Read the model definition and answer for the solid it produces. Units are mm, in the model's axes. Give positions to 0.01 mm unless a question says otherwise; leave off trailing zeros. Order: outer loops, then holes, each group sorted by start corner. A loop starts at its lowest first (then second) coordinate and runs counter-clockwise, first axis right, second up. Notation, with made-up numbers: M -11,10.25 L 6,10.25 A33 ccw 6,45.25 Z; hole C 68.5,-2.75 d8. An arc over 180 degrees is marked long. Write item = value, one per line. Start each with the question number.
from build123d import *

# Parameters (mm, degrees)
CROQUIS1_R              = 29.5
CROQUIS1_W              = 10
CROQUIS1_H              = 3
SALIENTE_EXTRUIR1_DEPTH = 3


with BuildPart() as part:
    # Croquis1 → Saliente-Extruir1 (new body)
    with BuildSketch(Plane(origin=(0, 0, 0), x_dir=(0, 0, -1), z_dir=(1, 0, 0))):
        with BuildLine():
            Line((-60, -82), (-40, -82))
            Line((-40, -82), (-40, -85))
            Line((-40, -85), (-20, -85))
            Line((-20, -85), (-20, -82))
            Line((-20, -82), (0, -82))
            Line((0, -82), (0, -85))
            Line((0, -85), (20, -85))
            Line((20, -85), (20, -82))
            Line((20, -82), (40, -82))
            Line((40, -82), (40, -85))
            Line((40, -85), (60, -85))
            Line((60, -85), (60, 25))
            ThreePointArc((60, 25), (0, 85), (-60, 25))
            Line((-60, 25), (-60, -82))
        make_face()
        with Locations((0, 25)):
            Circle(CROQUIS1_R, mode=Mode.SUBTRACT)
        with Locations((15, -60.5)):
            Rectangle(CROQUIS1_W, CROQUIS1_H, mode=Mode.SUBTRACT)
    extrude(amount=SALIENTE_EXTRUIR1_DEPTH)


solid = part.part
1) Find section C-C on y = 35. Determine the outline of the cut face in (x, z), plus the area to 3 significant figures.
2) Find section D-D on y = 71. Determine the outline of the cut face in (x, z).
3) Each of these flat-tipped pins is pushed along its axis until it touches: P1, Ø1.5, axis at x = 2, z = -31.5, coming from the -Y side; P2, Ø0.9, axis at x = 1, y = -83.5, coming from the +Z side. Where does it stop, or does it pass through?
4) Find section B-B on z = -26.5. Determine the outline of the cut face in (x, y), plus the area to 3 significant figures.
5) Find the intervals of material crossed by probe 1 along Y at (x, z) = (2.3, -15); probe 2 along Y at (x, z) = (0.7, -6.5); probe 3 along Y at (x, z) = (2, -2), in increasing order. Write a range as [from, to].
6) Find section A-A on x = 1.55. Determine the outline of the cut face in (y, z).
7) For a pull along Y with two mould halves and no side action, classify faces 1 (the face through (1.479, -3.799, 6.395)), 2 (the face through (3, -18, 1)), 3 (the face through (1.479, 84.985, -1.319)) as pulls with the +Y half, pulls with the -Y half, needs draft (parallel to the pull), parting line crosses it, or undercut.
Numbers:
q1.outline = M 0,-59.16 L 3,-59.16 L 3,-27.75 L 0,-27.75 Z; M 0,27.75 L 3,27.75 L 3,59.16 L 0,59.16 Z
q1.area = 188 mm2
q2.outline = M 0,-38.52 L 3,-38.52 L 3,38.52 L 0,38.52 Z
q3.P1 = -82
q3.P2 = 40
q4.outline = M 0,-82 L 3,-82 L 3,12.04 L 0,12.04 Z; M 0,37.96 L 3,37.96 L 3,78.83 L 0,78.83 Z
q4.area = 405 mm2
q5.probe_1 = [-85, -62], [-59, -0.4], [50.4, 83.09]
q5.probe_2 = [-85, -3.77], [53.77, 84.65]
q5.probe_3 = [-85, -4.43], [54.43, 84.97]
q6.outline = M -85,-60 L 25,-60 A60 ccw 25,60 L -82,60 L -82,40 L -85,40 L -85,20 L -82,20 L -82,0 L -85,0 L -85,-20 L -82,-20 L -82,-40 L -85,-40 Z; hole M -62,-20 L -59,-20 L -59,-10 L -62,-10 Z; hole C 25,0 d59
q7.face_1 = undercut
q7.face_2 = needs draft
q7.face_3 = pulls with the +Y half
